Autodesk Inventor part; units mm, degrees
ref_plane "YZ Plane" through (0, 0, 0) normal (1, 0, 0) x (0, 1, 0)
ref_plane "XZ Plane" through (0, 0, 0) normal (0, 1, 0) x (-1, 0, 0)
ref_plane "XY Plane" through (0, 0, 0) normal (0, 0, 1) x (1, 0, 0)
sketch "スケッチ1" plane through (0, 0, 0) normal (0, 0, 1) x (1, 0, 0)
  line L0 (0, 2.3094) -> (2, 1.1547)
  line L1 (2, 1.1547) -> (2, -1.1547)
  line L2 (2, -1.1547) -> (0, -2.3094)
  line L3 (0, -2.3094) -> (-2, -1.1547)
  line L4 (-2, -1.1547) -> (-2, 1.1547)
  line L5 (-2, 1.1547) -> (0, 2.3094)
  circle A0 centre (0, 0) radius 3.5
  line L6 (0, 0) -> (0, -20)
  circle A1 centre (0, -20) radius 2.5
  line L7 (2.5, -20) -> (2.5, -2.4495)
  line L8 (-2.5, -20) -> (-2.5, -2.4495)
  line L9 (-2, 1.1547) -> (-3.4875, 0.2959)
  line L10 (2, 1.1547) -> (3.4875, 0.2959)
  circle A2 centre (0, -2.3094) radius 4.6188
  line L11 (2, 1.1547) -> (2, 1.8539)
  line L12 (-2, 1.1547) -> (-2, 1.8539)
  dimension "d0" = 4
  dimension "d1" = 7
  dimension "d2" = 20
  dimension "d3" = 5
extrude "押し出し1" add sketch "スケッチ1" along normal blind 1.5 contours L10 A0 L6 L2 L1 | L11 A2 A0 L10 | L4 L3 L6 A0 L9 | L9 A0 A2 L12 | A0 A2 L7 | A0 L8 A2 | A0 L6 A2 L8 | A2 L6 A1 L8 | A0 L7 A2 L6 | L7 A1 L6 A2 | A1
fillet "フィレット1" radius 0.3 2 edges at (-2, 1.8539, 0.75) (2, 1.8539, 0.75)
fillet "フィレット2" radius 0.5 3 edges at (2, -1.1547, 0.75) (0, -2.3094, 0.75) (-2, -1.1547, 0.75)
fillet "フィレット3" radius 2 2 edges at (-2.5, -6.1931, 0.75) (2.5, -6.1931, 0.75)
properties part number "M2ナットレンチ"
Design review of the part built by this model. Coordinates are the model's own, in mm. A direction names the side the tool comes from. Give positions to 0.01 mm unless a question says otherwise; leave off trailing zeros. Loops run counter-clockwise (first coordinate to the right, second up) from the corner with the lowest first, then second, coordinate; pieces in that order, holes last. Notation, with made-up numbers: M 82.5,5.5 L 119.5,5.5 A11 cw 119.5,21.5 Z; hole C 81,61.25 d8. An arc over 180 degrees is marked long. One line per question, with ' | ' between items. Start each with the question number.
1. To check wall thickness, follow L1, parallel to Y at x = -4, z = 1.1; L2, parallel to X at y = -13.5, z = 0.8; L3, parallel to Y at x = 0, z = 0.5. State the ranges of each line that lie inside material, in increasing order.
2. Insertion check: P1, Ø0.8, axis at y = -13, z = 0.5, coming from the +X side. The pin has a flat end and moves straight along its axis. Give the tip position at first contact, or say it passes through.
3. Add section B-B (y = -1.75). Write out the cut boundary in (x, z).
4. Add section D-D (y = -14.5). Write out the cut boundary in (x, z), plus the area to 3 significant figures.
5. For faces 1 (the face through (-2.5, -14, 1)), 2 (the face through (2.5, -14, 1)), 3 (the face through (1.01, -1.726, 0.74)), 4 (the face through (0.1, -22.5, 0.7)), list the 3-axis set-ups (+Z, -Z, +X, -X, +Y, -Y) from which the entire face can be reached by the end or side of a thin tool; tool diameter is ignored.
6. The part is to be moulded in two halves that separate along X. For faces 5 (the face through (4.593, -1.822, 0.74)), 6 (the face through (-2, 0, 1)), 7 (the face through (-4.6, -1.9, 0.7)), say which applies: released by +X, released by -X, zero draft, split by the parting line, or undercut.
7. Add section A-A (z = 1.15). Write out the cut boundary in (x, y), plus the area to 3 significant figures.
8. Add section C-C (x = 0). Write out the cut boundary in (y, z).
Worked out:
1) L1: y = -4.62 to 0 | L2: x = -2.5 to 2.5 | L3: y = -22.5 to -2.23
2) P1: stops at x = 2.5
3) outline: M -4.58,0 L -0.97,0 L -0.97,1.5 L -4.58,1.5 Z; M 0.97,0 L 4.58,0 L 4.58,1.5 L 0.97,1.5 Z
4) outline: M -2.5,0 L 2.5,0 L 2.5,1.5 L -2.5,1.5 Z | area: 7.50 mm²
5) face 1: +Z, -Z, -X, -Y | face 2: +Z, -Z, +X, -Y | face 3: +Z, -Z, +Y | face 4: +Z, -Z, -Y
6) face 5: released by +X | face 6: undercut | face 7: released by -X
7) outline: M -3.14,-5.7 A2 cw -2.5,-7.16 L -2.5,-20 A2.5 ccw 2.5,-20 L 2.5,-7.16 A2 cw 3.14,-5.7 A4.62 ccw 2.46,1.6 A0.3 ccw 2,1.35 L 2,-0.87 A0.5 cw 1.75,-1.3 L 0.25,-2.17 A0.5 cw -0.25,-2.17 L -1.75,-1.3 A0.5 cw -2,-0.87 L -2,1.35 A0.3 ccw -2.46,1.6 A4.62 ccw Z | area: 128 mm²
8) outline: M -22.5,0 L -2.23,0 L -2.23,1.5 L -22.5,1.5 Z
